The model under review builds one solid part; all positions refer to its coordinate system, in mm. A direction names the side the tool comes from. Round coordinates to 2 decimals unless told otherwise and drop trailing zeros. Order: outer loops, then holes, each group sorted by start corner. A loop starts at its lowest first (then second) coordinate and runs counter-clockwise, first axis right, second up. Notation, with made-up numbers: (-18, 53) -> (-13, 53) arc R21 ccw to (-13, 59) -> close; hole circle Ø1 at (-34.5, -15). An arc over 180 degrees is marked (long way). Use a Markdown table: item, result. Add a question column.
```python
from build123d import *

# Parameters (mm, degrees)
BOX_W        = 16
BOX_H        = 14
BOX_DEPTH    = 15
BOX001_W     = 10
BOX001_H     = 10
BOX001_DEPTH = 20


with BuildPart() as cub:
    # Box → Box (new body)
    with BuildSketch(Plane.XY):
        with Locations((8, 7)):
            Rectangle(BOX_W, BOX_H)
    extrude(amount=BOX_DEPTH)


with BuildPart() as fusion:
    # Box001 → Box001 (new body)
    with BuildSketch(Plane(origin=(10, 0, 0), x_dir=(1, 0, 0), z_dir=(0, 0, 1))):
        with Locations((5, 5)):
            Rectangle(BOX001_W, BOX001_H)
    extrude(amount=BOX001_DEPTH)

    # Fusion: union Cub
    add(cub.part)


solid = fusion.part
```
Q1. Add section C-C (x = 18.75). Write out the cut boundary in (y, z), then the cut area to 3 significant figures.
Q2. Add section A-A (y = 5.5). Write out the cut boundary in (x, z).
Q3. Wall thickness on line 1 (X direction, y = 7.5, z = 18.25); line 2 (Z direction, x = 8.5, y = 5); line 3 (X direction, y = 13.75, z = 11.75): over which ranges is each line inside the solid? List them lowest first. Write a range as [from, to].
Q4. Add section D-D (y = 11.75). Write out the cut boundary in (x, z).
Q5. Machinability: for faces 1 (the flat face through (10, 5, 17)), 2 (the flat face through (0, 7, 7)), 3 (the flat face through (16, 12, 7)), which of the approach directions +Z, -Z, +X, -X, +Y, -Y give a long, thin tool a straight path to every point of the face, cutting with its end or side? Answer none if there is none.
Q6. Add section B-B (z = 13.25). Write out the cut boundary in (x, y), then the cut area to 3 significant figures.
Report:
| question | item | result |
|---|---|---|
| 1 | outline | (0, 0) -> (10, 0) -> (10, 20) -> (0, 20) -> close |
| 1 | area | 200 mm² |
| 2 | outline | (0, 0) -> (20, 0) -> (20, 20) -> (10, 20) -> (10, 15) -> (0, 15) -> close |
| 3 | line 1 | x = [10, 20] |
| 3 | line 2 | z = [0, 15] |
| 3 | line 3 | x = [0, 16] |
| 4 | outline | (0, 0) -> (16, 0) -> (16, 15) -> (0, 15) -> close |
| 5 | face 1 | +Z, -X, +Y, -Y |
| 5 | face 2 | +Z, -Z, -X, +Y, -Y |
| 5 | face 3 | +Z, -Z, +X, +Y |
| 6 | outline | (0, 0) -> (20, 0) -> (20, 10) -> (16, 10) -> (16, 14) -> (0, 14) -> close |
| 6 | area | 264 mm² |
